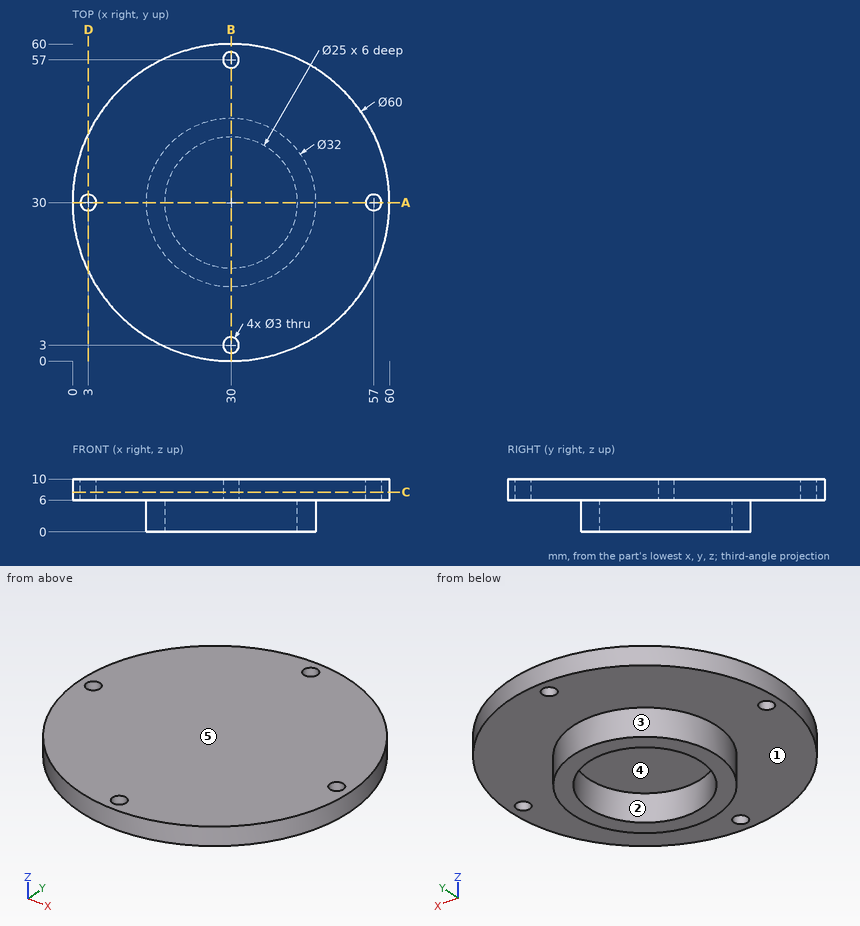
The drawing under review shows one solid part. Ordinate dimensions are in mm from its lowest x, y, z. A direction names the side the tool comes from. Coordinates: 2 decimals unless noted, no trailing zeros. Write each loop counter-clockwise with the first axis right and the second up, starting at its lowest first coordinate (ties: lowest second). Pieces come first, ordered by that corner, then holes. Notation, with made-up numbers: (55, -16.75) -> (81, -16.75) arc R27 ccw to (81, 13.25) -> close; hole circle Ø5 at (71.5, -1.5). An arc over 180 degrees is marked (long way). Write each question's results on one line, items separated by ' | '. Start each with the question number.
1) The part is to be moulded in two halves that separate along X. For the marked faces 1, 2 and 3, say which applies: +X half, -X half, draft (parallel to the pull), parting line (faces both ways), or undercut.
2) Consider section D-D (x = 3). Write out the cut boundary in (y, z).
3) Wall thickness on L1, parallel to Y at x = 30, z = 7.8; L2, parallel to Z at x = 25.5, y = 13; L3, parallel to Y at x = 34, z = 0.5: over which ranges is each line inside the solid? List them lowest first. Write a range as [from, to].
4) Consider section C-C (z = 7.5). Write out the cut boundary in (x, y), plus the area to 3 significant figures.
5) Consider section A-A (y = 30). Write out the cut boundary in (x, z), plus the area to 3 significant figures.
6) Insertion check: pin 1 (15 mm diameter, centred on x = 30, y = 30, fed in from -Z); pin 2 (1 mm diameter, centred on y = 15, z = 5, fed in from -X); pin 3 (3 mm diameter, centred on x = 39, z = 1, fed in from +Y). Each pin has a flat end and moves straight along its axis. Give the tip position at first contact, or say it passes through.
7) For the marked faces 4 and 5, list the 3-axis set-ups (+Z, -Z, +X, -X, +Y, -Y) from which the entire face can be reached by the end or side of a thin tool; tool diameter is ignored.
Geometry says:
1) face 1: draft | face 2: undercut | face 3: parting line
2) outline: (16.92, 6) -> (28.5, 6) -> (28.5, 10) -> (16.92, 10) -> close; (31.5, 6) -> (43.08, 6) -> (43.08, 10) -> (31.5, 10) -> close
3) L1: [0, 1.5], [4.5, 55.5], [58.5, 60] | L2: [6, 10] | L3: [14.51, 18.16], [41.84, 45.49]
4) outline: circle Ø60 at (30, 30); hole circle Ø3 at (3, 30); hole circle Ø3 at (30, 3); hole circle Ø3 at (30, 57); hole circle Ø3 at (57, 30) | area: 2,800 mm^2
5) outline: (0, 6) -> (1.5, 6) -> (1.5, 10) -> (0, 10) -> close; (4.5, 6) -> (14, 6) -> (14, 0) -> (17.5, 0) -> (17.5, 6) -> (42.5, 6) -> (42.5, 0) -> (46, 0) -> (46, 6) -> (55.5, 6) -> (55.5, 10) -> (4.5, 10) -> close; (58.5, 6) -> (60, 6) -> (60, 10) -> (58.5, 10) -> close | area: 258 mm^2
6) pin 1: z = 6 | pin 2: x = 23.24 | pin 3: y = 44.13
7) face 4: -Z | face 5: +Z, +X, -X, +Y, -Y
